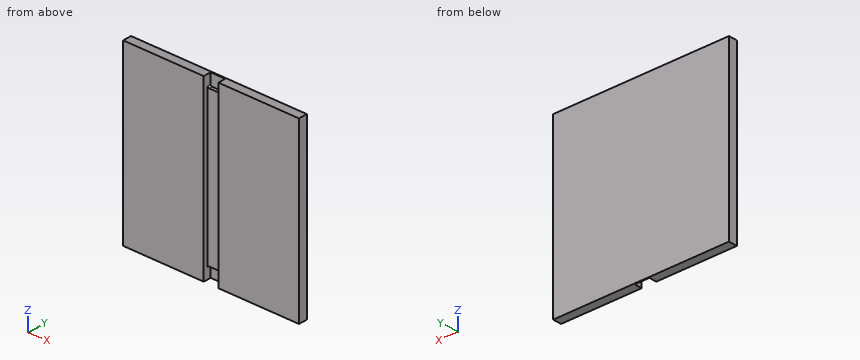
```python
from build123d import *

# Parameters (mm, degrees)
F0_W     = 174.625
F0_H     = 381
F1_DEPTH = 12.7
F0_W_2   = 31.75
F2_DEPTH = 3.175
F4_W     = 381
F4_H     = 381
F5_DEPTH = 6.35
F6_DEPTH = 16.66875


with BuildPart() as f1:
    # F0 (on Front) → F1 (new body)
    with BuildSketch(Plane.XZ):
        with Locations((-111.50095, 51.705398)):
            Rectangle(F0_W, F0_H)
        with Locations((94.87405, 51.705398)):
            Rectangle(F0_W, F0_H)
    extrude(amount=F1_DEPTH)

    # F0 (on Front) → F2 (join)
    with BuildSketch(Plane.XZ):
        with Locations((-8.31345, 51.705398)):
            Rectangle(F0_W_2, F0_H)
    extrude(amount=F2_DEPTH)

    # F4 (on face) → F5 (join)
    with BuildSketch(Plane.XZ):
        with Locations((-8.31345, 51.705398)):
            Rectangle(F4_W, F4_H)
    extrude(amount=-F5_DEPTH)

    # F3 (on face) → F6 (cut)
    with BuildSketch(Plane.XZ.offset(12.7)):
        with BuildLine():
            Line((-24.18845, -116.569602), (-24.18845, -138.794602))
            Line((-24.18845, -138.794602), (7.56155, -138.794602))
            Line((7.56155, -138.794602), (7.56155, -116.569602))
            ThreePointArc((7.56155, -116.569602), (6.631614, -114.324538), (4.38655, -113.394602))
            Line((4.38655, -113.394602), (-21.01345, -113.394602))
            ThreePointArc((-21.01345, -113.394602), (-23.258514, -114.324538), (-24.18845, -116.569602))
        make_face()
        with BuildLine():
            ThreePointArc((-24.18845, 219.980398), (-23.258514, 217.735334), (-21.01345, 216.805398))
            Line((-21.01345, 216.805398), (4.38655, 216.805398))
            ThreePointArc((4.38655, 216.805398), (6.631614, 217.735334), (7.56155, 219.980398))
            Line((7.56155, 219.980398), (7.56155, 242.205398))
            Line((7.56155, 242.205398), (-24.18845, 242.205398))
            Line((-24.18845, 242.205398), (-24.18845, 219.980398))
        make_face()
    extrude(amount=-F6_DEPTH, mode=Mode.SUBTRACT)


solid = f1.part
```
CAD build for the part. Positions are in the model's coordinates, mm. Round coordinates to 2 decimals unless told otherwise and drop trailing zeros. Loops run counter-clockwise (first coordinate to the right, second up) from the corner with the lowest first, then second, coordinate; pieces in that order, holes last. Notation, with made-up numbers: (47, 57) - (91, 57) arc R4 cw to (91, 64) - close; hole circle Ø8 at (65.5, 17.5). An arc over 180 degrees is marked (long way). Return JSON: item names as keys, results as strings. Group by question number.
Q1. Drill centre lines: line 1 along X through (y, z) = (-12, 49.5); line 2 along Z through (x, y) = (2, 3.75). Where is each one in solid material? Low to high. Write a range as [from, to].
Q2. Band-saw the part on A-A on y = -8. Give the cut face in (x, z).
Q3. Flat gauge pins, fed straight in: pin 1 Ø9.5 at (x, z) = (-5.5, 60.5) entering from -Y (3 decimals); pin 2 Ø20.5 at (x, z) = (-6, -127) entering from -Y; pin 3 Ø3.5 at (x, y) = (-6, -0.5) entering from +Z. Where does each tip first touch, or does it go through?
Q4. Band-saw the part on B-B on z = -19. Give the cut face in (x, y) (3 decimals).
Solutions:
{
 "1": {"line 1": "x = [-198.81, -24.19], [7.56, 182.19]", "line 2": "z = [-113.39, 216.81]"},
 "2": {"outline": "(-198.81, -138.79) - (-24.19, -138.79) - (-24.19, 242.21) - (-198.81, 242.21) - close; (7.56, -138.79) - (182.19, -138.79) - (182.19, 242.21) - (7.56, 242.21) - close"},
 "3": {"pin 1": "stops at y = -3.175", "pin 2": "stops at y = 3.97", "pin 3": "stops at z = 216.81"},
 "4": {"outline": "(-198.813, -12.7) - (-24.188, -12.7) - (-24.188, -3.175) - (7.562, -3.175) - (7.562, -12.7) - (182.187, -12.7) - (182.187, 6.35) - (-198.813, 6.35) - close"}
}
